Design review of the part built by this model. Coordinates are the model's own, in mm. Face numbers are marked on the shaded views. A direction names the side the tool comes from. Give positions to 0.01 mm unless a question says otherwise; leave off trailing zeros. Write each loop counter-clockwise with the first axis right and the second up, starting at its lowest first coordinate (ties: lowest second). Pieces come first, ordered by that corner, then holes. Notation, with made-up numbers: (-11.5, -9) -> (44.5, -9) arc R21 ccw to (44.5, 22) -> close; hole circle Ø1 at (-17, -30.75). An arc over 180 degrees is marked (long way). Answer as a JSON object with one key per item and string values.
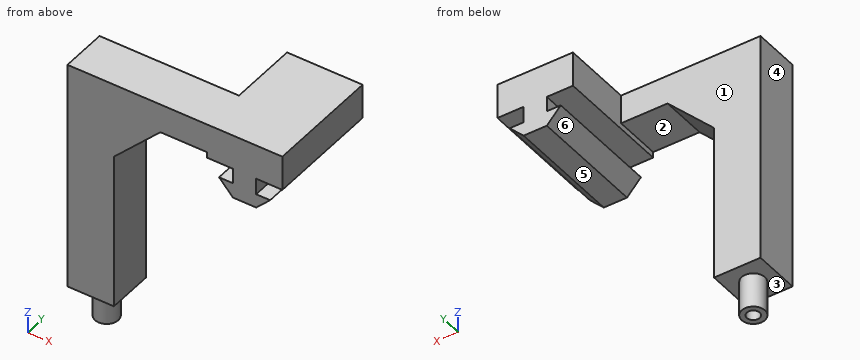
Autodesk Inventor part; units mm, degrees
ref_plane "YZ Plane" through (0, 0, 0) normal (1, 0, 0) x (0, 1, 0)
ref_plane "XZ Plane" through (0, 0, 0) normal (0, 1, 0) x (-1, 0, 0)
ref_plane "XY Plane" through (0, 0, 0) normal (0, 0, 1) x (1, 0, 0)
sketch "Sketch1" plane through (0, 0, 0) normal (0, 1, 0) x (-1, 0, 0)
  line L0 (0, 0) -> (16.51, 0)
  line L1 (16.51, 0) -> (16.51, 7.62)
  line L2 (16.51, 7.62) -> (0, 7.62)
  line L3 (0, 7.62) -> (0, 0)
  line L4 (16.51, 0) -> (10.795, 0)
  line L5 (10.795, 0) -> (10.795, -6.604)
  line L6 (10.795, -6.604) -> (5.715, -6.604)
  line L7 (5.715, -6.604) -> (5.715, 0)
  line L8 (5.715, -6.604) -> (5.715, -3.556)
  line L9 (5.715, -3.556) -> (2.667, -3.556)
  line L10 (2.667, -3.556) -> (5.715, -6.604)
  line L11 (10.795, -3.302) -> (13.843, -3.302)
  line L12 (13.843, -3.302) -> (10.795, -6.604)
  dimension "d0" = 16.51
  dimension "d1" = 7.62
  dimension "d2" = 5.715
  dimension "d3" = 6.604
  dimension "d4" = 5.08
  dimension "d5" = 3.048
  dimension "d6" = 3.048
  dimension "d7" = 3.048
extrude "Extrusion1" add sketch "Sketch1" along normal blind 25.4
sketch "Sketch3" plane through (-16.51, 0, 0) normal (-1, 0, 0) x (0, 0, 1)
  line L0 (0, 0) -> (7.62, 0)
  line L1 (7.62, 0) -> (1.27, 0)
  line L2 (1.27, 0) -> (1.27, 10.16)
  line L3 (1.27, 10.16) -> (7.62, 10.16)
  line L4 (7.62, 10.16) -> (7.62, 0)
  dimension "d10" = 6.35
  dimension "d11" = 10.16
extrude "Extrusion2" add sketch "Sketch3" along normal blind 30.48
sketch "Sketch4" plane through (-16.51, 0, 1.27) normal (0, 0, -1) x (-1, 0, 0)
  line L0 (30.48, 10.16) -> (30.48, 0)
  line L1 (30.48, 10.16) -> (20.32, 10.16)
  line L2 (20.32, 10.16) -> (20.32, 0)
  line L3 (20.32, 0) -> (30.48, 0)
  line L4 (30.48, 0) -> (30.48, 10.16)
  point P0 (-16.51, 0)
  dimension "d14" = 10.16
  dimension "d15" = 10.16
extrude "Extrusion3" add sketch "Sketch4" along normal blind 44.45
sketch "Sketch5" plane through (-16.51, 0, -43.18) normal (0, 0, -1) x (-1, 0, 0)
  line L0 (30.48, 0) -> (30.48, 10.16)
  line L1 (30.48, 5.08) -> (25.4, 5.08)
  circle A0 centre (25.4, 5.08) radius 2.54
  point P0 (-16.51, 0)
  dimension "d18" = 5.08
  dimension "d19" = 5.08
extrude "Extrusion4" add sketch "Sketch5" along normal blind 7.62
sketch "Sketch6" plane through (-41.91, 5.08, -50.8) normal (0, 0, -1) x (-1, 0, 0)
  circle A0 centre (0, 0) radius 2.54
  line L0 (2.54, 0) -> (0, 0)
  point P0 (-41.91, -5.08)
hole "Hole1" at (-41.91, 5.08, -50.8) direction (0, 0, 1) diameter 2.794 depth 16.002 tip angle 118
sketch "Sketch7" plane through (-16.51, 0, 1.27) normal (0, 0, -1) x (-1, 0, 0)
  line L0 (20.32, 0) -> (20.32, 10.16)
  line L1 (0, 0) -> (20.32, 0)
  line L2 (20.32, 10.16) -> (10.16, 10.16)
  line L3 (10.16, 10.16) -> (10.16, 0)
  line L4 (10.16, 0) -> (20.32, 0)
  line L5 (20.32, 0) -> (20.32, 10.16)
  point P0 (-16.51, 0)
  dimension "d29" = 10.16
extrude "Extrusion5" add sketch "Sketch7" along normal blind 10.16
chamfer "Chamfer1" distance 10.16 angle 45 1 edges at (-26.67, 5.08, -8.89)
properties part number "Grab Rail v2.5 - Left"
(1) The part is to be moulded in two halves that separate along X. For the marked faces 4, 5 and 6, say which applies: +X half, -X half, draft (parallel to the pull), parting line (faces both ways), or undercut.
Here are the results:
{"face 4": "-X half", "face 5": "draft", "face 6": "undercut"}
(2) We need section B-B, the plane x = -37.5. State the section outline as (y, z) points.
Here are the results:
{"outline": "(0, -43.18) -> (10.16, -43.18) -> (10.16, 7.62) -> (0, 7.62) -> close"}
(3) For the marked faces 1, 2 and 3, list the 3-axis set-ups (+Z, -Z, +X, -X, +Y, -Y) from which the entire face can be reached by the end or side of a thin tool; tool diameter is ignored.
Here are the results:
{"face 1": "+Z, -Z, -X, +Y", "face 2": "-Z, +Y, -Y", "face 3": "-Z"}
(4) We need section C-C, the plane y = 15.5. State the section outline as (x, z) points (3 decimals).
Here are the results:
{"outline": "(-16.51, 0) -> (-10.795, 0) -> (-10.795, -3.302) -> (-13.843, -3.302) -> (-10.795, -6.604) -> (-5.715, -6.604) -> (-2.667, -3.556) -> (-5.715, -3.556) -> (-5.715, 0) -> (0, 0) -> (0, 7.62) -> (-16.51, 7.62) -> close"}
(5) For line 1 along Y through (x, z) = (-41.91, -45); line 2 along Y through (x, z) = (-41.91, -40); line 3 along Z through (x, y) = (-8, 18), list the stretches that pass through material, from the lowest coordinate up.
Here are the results:
{"line 1": "y = 2.54 to 3.68, 6.48 to 7.62", "line 2": "y = 0 to 3.68, 6.48 to 10.16", "line 3": "z = -6.6 to 7.62"}
(6) Clearance check with flat-ended pins moving along their axes: pin 1 (15 mm diameter, centred on x = -27.5, z = -11, fed in from +Y); pin 2 (12 mm diameter, centred on y = 6.5, z = -38.5, fed in from +X); pin 3 (4.5 mm diameter, centred on x = -3.5, y = 16, fed in from -Z); pin 4 (1.7 mm diameter, centred on x = -13, y = 8.5, fed in from -Z). State where each tip first meets the part, or that it passes through.
Here are the results:
{"pin 1": "passes through", "pin 2": "stops at x = -36.83", "pin 3": "stops at z = -6.6", "pin 4": "stops at z = -5.14"}
(7) We need section D-D, the plane z = -30. State the section outline as (x, y) points.
Here are the results:
{"outline": "(-46.99, 0) -> (-36.83, 0) -> (-36.83, 10.16) -> (-46.99, 10.16) -> close"}
